```python
from build123d import *

# Parameters (mm, degrees)
SKETCH1_W           = 4.3434
SKETCH1_H           = 27.20594
BOSS_EXTRUDE1_DEPTH = 1.6002
FILLET1_R           = 0.508
FILLET2_R           = 0.508
FILLET3_R           = 0.254


with BuildPart() as part:
    # Sketch1 → Boss-Extrude1 (new body)
    with BuildSketch(Plane.XY):
        with BuildLine():
            Line((0, 51.4198), (-6.02742, 51.103916303))
            Line((-6.02742, 51.103916303), (-6.02742, 21.146463697))
            Line((-6.02742, 21.146463697), (0, 20.83058))
            Line((0, 20.83058), (0, 20.24638))
            Line((0, 20.24638), (-5.08, 19.53243256))
            Line((-5.08, 19.53243256), (-5.08, 9.19504744))
            Line((-5.08, 9.19504744), (0, 8.4811))
            Line((0, 8.4811), (0, 5.334))
            ThreePointArc((0, 5.334), (1.562292429, 1.562292429), (5.334, 0))
            Line((5.334, 0), (55.64639368, 0))
            ThreePointArc((55.64639368, 0), (59.220505665, 1.374545553), (60.952555507, 4.789754962))
            ThreePointArc((60.952555507, 4.789754962), (62.542276693, 35.823920719), (60.961816866, 66.858559503))
            ThreePointArc((60.961816866, 66.858559503), (59.230195601, 70.274819072), (55.65549286, 71.649897966))
            Line((55.65549286, 71.649897966), (5.334, 71.649897966))
            ThreePointArc((5.334, 71.649897966), (1.562292429, 70.087605537), (0, 66.315897966))
            Line((0, 66.315897966), (0, 51.4198))
        make_face()
        with BuildLine():
            Line((5.334, 70.125897966), (55.65549286, 70.125897966))
            ThreePointArc((55.65549286, 70.125897966), (58.208851961, 69.143698756), (59.445724293, 66.70351335))
            ThreePointArc((59.445724293, 66.70351335), (61.01827671, 35.824148117), (59.436509271, 4.945253544))
            ThreePointArc((59.436509271, 4.945253544), (58.199330812, 2.505818252), (55.64639368, 1.524))
            Line((55.64639368, 1.524), (5.334, 1.524))
            ThreePointArc((5.334, 1.524), (2.639923164, 2.639923164), (1.524, 5.334))
            Line((1.524, 5.334), (1.524, 66.315897966))
            ThreePointArc((1.524, 66.315897966), (2.639923164, 69.009974802), (5.334, 70.125897966))
        make_face(mode=Mode.SUBTRACT)
        with Locations((-2.2987, 36.12519)):
            Rectangle(SKETCH1_W, SKETCH1_H, mode=Mode.SUBTRACT)
        Polygon((-0.8382, 18.35662), (-3.70332, 18.35662), (-3.70332, 10.3734), (-0.8382, 10.3734), (-0.8382, 9.9924), (-0.0762, 9.9924), (-0.0762, 18.73762), (-0.8382, 18.73762), align=None, mode=Mode.SUBTRACT)
    extrude(amount=BOSS_EXTRUDE1_DEPTH)

    # Fillet1
    fillet1_edges = [part.edges().sort_by_distance(p)[0] for p in [
        (-3.70332, 18.35662, 0.8001),
        (-3.70332, 10.3734, 0.8001),
    ]]
    fillet(fillet1_edges, radius=FILLET1_R)

    # Fillet2
    fillet2_edges = [part.edges().sort_by_distance(p)[0] for p in [
        (-5.08, 9.19504744, 0.8001),
        (-5.08, 19.53243256, 0.8001),
        (-6.02742, 21.146463697, 0.8001),
        (-6.02742, 51.103916303, 0.8001),
    ]]
    fillet(fillet2_edges, radius=FILLET2_R)

    # Fillet3
    fillet3_edges = [part.edges().sort_by_distance(p)[0] for p in [
        (0, 8.4811, 0.8001),
        (0, 20.24638, 0.8001),
        (0, 20.83058, 0.8001),
        (0, 51.4198, 0.8001),
        (-0.127, 22.52222, 0.8001),
        (-0.127, 49.72816, 0.8001),
        (-4.4704, 49.72816, 0.8001),
        (-4.4704, 22.52222, 0.8001),
        (-0.8382, 9.9924, 0.8001),
        (-0.0762, 9.9924, 0.8001),
        (-0.0762, 18.73762, 0.8001),
        (-0.8382, 18.73762, 0.8001),
    ]]
    fillet(fillet3_edges, radius=FILLET3_R)


solid = part.part
```
Read the model definition and answer for the solid it produces. Units are mm, in the model's axes. A direction names the side the tool comes from. Give positions to 0.01 mm unless a question says otherwise; leave off trailing zeros. Order: outer loops, then holes, each group sorted by start corner. A loop starts at its lowest first (then second) coordinate and runs counter-clockwise, first axis right, second up. Notation, with made-up numbers: (64, -23) -> (97, -23) arc R5 ccw to (97, -18) -> close; hole circle Ø11 at (65, -10.5). An arc over 180 degrees is marked (long way). One line per item, written item: value. Start each with the question number.
(1) A tool of negligible diameter and unlimited length cuts with its end or side. For faces 4 (the flat face through (0, 7, 1)), 5 (the flat face through (-2.4, 19.91, 0.79)), 6 (the flat face through (-0.076, 14, 1)), from which of +Z, -Z, +X, -X, +Y, -Y can it reach the whole face along a straight path? Write none if from no direction.
(2) For a pull along X with two mould halves and no side action, classify faces 1 (the cylindrical face through (59.27, 70.24, 0.79)), 2 (the cylindrical face through (61.02, 36.26, 0.79)), 3 (the flat face through (-2.462, 8.827, 0.789)) as released by +X, released by -X, zero draft, split by the parting line, or undercut.
(3) The part is cut by section B-B (y = 65). Determine the outline of the cut face in (x, z), and give its area (3 significant figures).
(4) The part is cut by section D-D (z = 0.9). State how many separate pieces and enclosed holes the cut face has, and give its area (3 significant figures).
(5) Flat-ended cylindrical pins translate along their axes: P1, Ø0.5, axis at x = -2, z = 1, coming from the +Y side; P2, Ø0.5, axis at x = -2.5, z = 0.5, coming from the -Y side; P3, Ø0.5, axis at x = -1.5, z = 0.5, coming from the -Y side. Find the tip coordinate at first contact, or state that the pin passes through.
(6) The part is cut by section A-A (x = 44). Determine the outline of the cut face in (y, z), and give its area (3 significant figures).
(7) The part is cut by section C-C (y = 40.5). Determine the outline of the cut face in (x, z).
(8) Straight lines are drawn through the part: L1, parallel to X at y = 41.5, z = 1.4; L2, parallel to X at y = 18.5, z = 0.2; L3, parallel to Y at x = 20, z = 1.35. For each, find the intervals that lie inside material, in ascending order.
Taken from the geometry:
1. face 4: +Z, -Z, -X, -Y
1. face 5: +Z, -Z, -X
1. face 6: +Z, -Z
2. face 1: released by +X
2. face 2: undercut
2. face 3: released by -X
3. outline: (0, 0) -> (1.52, 0) -> (1.52, 1.6) -> (0, 1.6) -> close; (59.62, 0) -> (61.15, 0) -> (61.15, 1.6) -> (59.62, 1.6) -> close
3. area: 4.89 mm^2
4. separate pieces: 1
4. enclosed holes: 3
4. area: 474 mm^2
5. P1: y = 51.33
5. P2: y = 8.8
5. P3: y = 8.66
6. outline: (0, 0) -> (1.52, 0) -> (1.52, 1.6) -> (0, 1.6) -> close; (70.13, 0) -> (71.65, 0) -> (71.65, 1.6) -> (70.13, 1.6) -> close
6. area: 4.88 mm^2
7. outline: (-6.03, 0) -> (-4.47, 0) -> (-4.47, 1.6) -> (-6.03, 1.6) -> close; (-0.13, 0) -> (1.52, 0) -> (1.52, 1.6) -> (-0.13, 1.6) -> close; (60.98, 0) -> (62.51, 0) -> (62.51, 1.6) -> (60.98, 1.6) -> close
8. L1: -6.03 to -4.47, -0.13 to 1.52, 60.97 to 62.49
8. L2: -5.08 to -0.84, -0.08 to 1.52, 60.52 to 62.05
8. L3: 0 to 1.52, 70.13 to 71.65
